```python
from build123d import *

# Parameters (mm, degrees)
SKETCH1_W           = 31.75
SKETCH1_H           = 31.75
BOSS_EXTRUDE1_DEPTH = 114.3
SKETCH3_W           = 24.13
SKETCH3_H           = 24.13
CUT_EXTRUDE1_DEPTH  = 114.3
SKETCH4_W           = 19.05
SKETCH4_H           = 25.4
CUT_EXTRUDE4_DEPTH  = 6.35
SKETCH10_W          = 25.4
SKETCH10_H          = 19.05
CUT_EXTRUDE5_DEPTH  = 6.35
SKETCH13_W          = 19.05
SKETCH13_H          = 25.4
CUT_EXTRUDE6_DEPTH  = 6.35
SKETCH14_W          = 25.4
SKETCH14_H          = 19.05
CUT_EXTRUDE7_DEPTH  = 6.35
FILLET1_64_R        = 0.396875


with BuildPart() as part:
    # Sketch1 → Boss-Extrude1 (new body)
    with BuildSketch(Plane.XY):
        with Locations((-6.389302447, 3.219010904)):
            Rectangle(SKETCH1_W, SKETCH1_H)
    extrude(amount=BOSS_EXTRUDE1_DEPTH)

    # Sketch3 → Cut-Extrude1 (cut)
    with BuildSketch(Plane.XY.offset(114.3)):
        with Locations((-6.389302447, 3.219010904)):
            Rectangle(SKETCH3_W, SKETCH3_H)
    extrude(amount=-CUT_EXTRUDE1_DEPTH, mode=Mode.SUBTRACT)

    # Sketch4 → Cut-Extrude4 (cut)
    with BuildSketch(Plane(origin=(0, 19.094010904, 0), x_dir=(1, 0, 0), z_dir=(0, 1, 0))):
        with Locations((-6.389302447, -76.2)):
            Rectangle(SKETCH4_W, SKETCH4_H)
        with Locations((-6.389302447, -38.1)):
            Rectangle(SKETCH4_W, SKETCH4_H)
    extrude(amount=-CUT_EXTRUDE4_DEPTH, mode=Mode.SUBTRACT)

    # Sketch10 → Cut-Extrude5 (cut)
    with BuildSketch(Plane(origin=(9.485697553, 0, 0), x_dir=(0, 0, -1), z_dir=(1, 0, 0))):
        with Locations((-76.2, 3.219010904)):
            Rectangle(SKETCH10_W, SKETCH10_H)
        with Locations((-38.1, 3.219010904)):
            Rectangle(SKETCH10_W, SKETCH10_H)
    extrude(amount=-CUT_EXTRUDE5_DEPTH, mode=Mode.SUBTRACT)

    # Sketch13 → Cut-Extrude6 (cut)
    with BuildSketch(Plane.XZ.offset(12.655989096)):
        with Locations((-6.389302447, 76.2)):
            Rectangle(SKETCH13_W, SKETCH13_H)
        with Locations((-6.389302447, 38.1)):
            Rectangle(SKETCH13_W, SKETCH13_H)
    extrude(amount=-CUT_EXTRUDE6_DEPTH, mode=Mode.SUBTRACT)

    # Sketch14 → Cut-Extrude7 (cut)
    with BuildSketch(Plane.ZY.offset(22.264302447)):
        with Locations((76.2, 3.219010904)):
            Rectangle(SKETCH14_W, SKETCH14_H)
        with Locations((38.1, 3.219010904)):
            Rectangle(SKETCH14_W, SKETCH14_H)
    extrude(amount=-CUT_EXTRUDE7_DEPTH, mode=Mode.SUBTRACT)

    # Fillet1/64
    fillet1_64_edges = [part.edges().sort_by_distance(p)[0] for p in [
        (-15.914302447, -8.845989096, 38.1),
        (-6.389302447, -8.845989096, 25.4),
        (3.135697553, -8.845989096, 38.1),
        (-6.389302447, -8.845989096, 50.8),
        (-6.389302447, -8.845989096, 63.5),
        (3.135697553, -8.845989096, 76.2),
        (-6.389302447, -8.845989096, 88.9),
        (-15.914302447, -8.845989096, 76.2),
        (-15.914302447, -12.655989096, 76.2),
        (-6.389302447, -12.655989096, 63.5),
        (3.135697553, -12.655989096, 76.2),
        (-6.389302447, -12.655989096, 88.9),
        (9.485697553, 3.219010904, 114.3),
        (-6.389302447, -12.655989096, 50.8),
        (-15.914302447, -12.655989096, 38.1),
        (-6.389302447, -12.655989096, 25.4),
        (3.135697553, -12.655989096, 38.1),
        (-18.454302447, 12.744010904, 38.1),
        (-18.454302447, 3.219010904, 25.4),
        (-18.454302447, -6.305989096, 38.1),
        (-18.454302447, 3.219010904, 50.8),
        (-18.454302447, 3.219010904, 63.5),
        (-18.454302447, -6.305989096, 76.2),
        (-18.454302447, 3.219010904, 88.9),
        (-18.454302447, 12.744010904, 76.2),
        (-22.264302447, 12.744010904, 76.2),
        (-22.264302447, 3.219010904, 63.5),
        (-22.264302447, -6.305989096, 76.2),
        (-22.264302447, 3.219010904, 88.9),
        (-6.389302447, 19.094010904, 114.3),
        (-22.264302447, 3.219010904, 50.8),
        (-22.264302447, 12.744010904, 38.1),
        (-22.264302447, 3.219010904, 25.4),
        (-22.264302447, -6.305989096, 38.1),
        (-6.389302447, -8.845989096, 0),
        (5.675697553, -8.845989096, 57.15),
        (-18.454302447, 3.219010904, 0),
        (-18.454302447, -8.845989096, 57.15),
        (-6.389302447, 15.284010904, 114.3),
        (-18.454302447, 15.284010904, 57.15),
        (5.675697553, 3.219010904, 114.3),
        (5.675697553, 15.284010904, 57.15),
        (-6.389302447, 15.284010904, 0),
        (5.675697553, 3.219010904, 0),
        (-6.389302447, -8.845989096, 114.3),
        (-18.454302447, 3.219010904, 114.3),
        (-6.389302447, 15.284010904, 50.8),
        (3.135697553, 15.284010904, 38.1),
        (-6.389302447, 15.284010904, 25.4),
        (-15.914302447, 15.284010904, 38.1),
        (3.135697553, 15.284010904, 76.2),
        (-6.389302447, 15.284010904, 63.5),
        (-15.914302447, 15.284010904, 76.2),
        (-6.389302447, 15.284010904, 88.9),
        (-15.914302447, 19.094010904, 76.2),
        (-6.389302447, 19.094010904, 63.5),
        (-6.389302447, 19.094010904, 88.9),
        (3.135697553, 19.094010904, 76.2),
        (-6.389302447, 19.094010904, 25.4),
        (3.135697553, 19.094010904, 38.1),
        (-15.914302447, 19.094010904, 38.1),
        (-6.389302447, 19.094010904, 50.8),
        (-22.264302447, 3.219010904, 114.3),
        (-6.389302447, 19.094010904, 0),
        (9.485697553, 3.219010904, 0),
        (-6.389302447, -12.655989096, 0),
        (-22.264302447, 3.219010904, 0),
        (5.675697553, 12.744010904, 38.1),
        (5.675697553, 3.219010904, 50.8),
        (5.675697553, -6.305989096, 38.1),
        (5.675697553, 3.219010904, 25.4),
        (5.675697553, -6.305989096, 76.2),
        (5.675697553, 3.219010904, 63.5),
        (5.675697553, 12.744010904, 76.2),
        (5.675697553, 3.219010904, 88.9),
        (-22.264302447, 19.094010904, 57.15),
        (9.485697553, 12.744010904, 76.2),
        (9.485697553, 19.094010904, 57.15),
        (9.485697553, 3.219010904, 63.5),
        (9.485697553, -12.655989096, 57.15),
        (9.485697553, 3.219010904, 88.9),
        (9.485697553, -6.305989096, 76.2),
        (-22.264302447, -12.655989096, 57.15),
        (9.485697553, 3.219010904, 25.4),
        (9.485697553, -6.305989096, 38.1),
        (-6.389302447, -12.655989096, 114.3),
        (9.485697553, 12.744010904, 38.1),
        (9.485697553, 3.219010904, 50.8),
    ]]
    fillet(fillet1_64_edges, radius=FILLET1_64_R)


solid = part.part
```
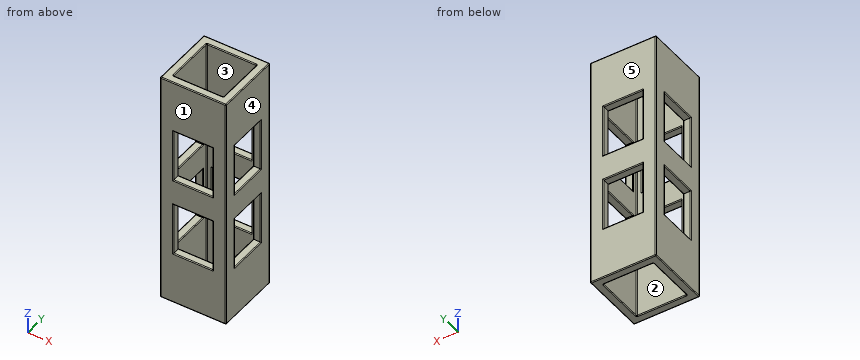
Read the model definition and answer for the solid it produces. Units are mm, in the model's axes. Face numbers are marked on the shaded views. A direction names the side the tool comes from. Round coordinates to 2 decimals unless told otherwise and drop trailing zeros. Write each loop counter-clockwise with the first axis right and the second up, starting at its lowest first coordinate (ties: lowest second). Pieces come first, ordered by that corner, then holes. Notation, with made-up numbers: M -9,-7 L 42,-7 A16 ccw 42,3 Z; hole C 36.25,27.25 d10. An arc over 180 degrees is marked long. One line per item, written item: value.
Q1. Straight lines are drawn through the part: line 1 (Z direction, x = -10, y = -10.5); line 2 (Y direction, x = -18, z = 21); line 3 (X direction, y = 17, z = 75). For each, find the intervals that lie inside material, in ascending order. Write a range as [from, to].
Data:
line 1: [0, 25.4], [50.8, 63.5], [88.9, 114.3]
line 2: [-12.66, -8.85], [15.28, 19.09]
line 3: [-22.26, -15.91], [3.14, 9.49]
Q2. Find section C-C on z = 99. Write down the section's boundary in (x, y).
Data:
outline: M -22.26,-12.26 A0.4 ccw -21.87,-12.66 L 9.09,-12.66 A0.4 ccw 9.49,-12.26 L 9.49,18.7 A0.4 ccw 9.09,19.09 L -21.87,19.09 A0.4 ccw -22.26,18.7 Z; hole M -18.45,-8.45 A0.4 ccw -18.06,-8.85 L 5.28,-8.85 A0.4 ccw 5.68,-8.45 L 5.68,14.89 A0.4 ccw 5.28,15.28 L -18.06,15.28 A0.4 ccw -18.45,14.89 Z
Q3. For a pull along Y with two mould halves and no side action, classify the marked faces 3, 4 and 5 as +Y half, -Y half, draft (parallel to the pull), parting line (faces both ways), or undercut.
Data:
face 3: undercut
face 4: draft
face 5: +Y half
Q4. Which of the six approach directions +Z, -Z, +X, -X, +Y, -Y give full straight-line access (tool end or side, diameter ignored) to the marked faces 1 and 2?
Data:
face 1: +Z, -Z, +X, -X, -Y
face 2: +Z, -Z
Q5. Find section D-D on y = -4.5. Count the separate pieces of the cut face and the enclosed holes in it, plus the area to 3 significant figures.
Data:
separate pieces: 6
enclosed holes: 0
area: 483 mm2
Q6. Find section B-B on y = 17. Write down the section's boundary in (x, z), plus the area to 3 significant figures.
Data:
outline: M -22.26,0.4 A0.4 ccw -21.87,0 L 9.09,0 A0.4 ccw 9.49,0.4 L 9.49,113.9 A0.4 ccw 9.09,114.3 L -21.87,114.3 A0.4 ccw -22.26,113.9 Z; hole M -15.91,25.4 L 3.14,25.4 L 3.14,50.8 L -15.91,50.8 Z; hole M -15.91,63.5 L 3.14,63.5 L 3.14,88.9 L -15.91,88.9 Z
area: 2,660 mm2
Q7. Find section A-A on x = 7.5. Write down the section's boundary in (y, z).
Data:
outline: M -12.66,0.4 A0.4 ccw -12.26,0 L 18.7,0 A0.4 ccw 19.09,0.4 L 19.09,113.9 A0.4 ccw 18.7,114.3 L -12.26,114.3 A0.4 ccw -12.66,113.9 Z; hole M -6.31,25.4 L 12.74,25.4 L 12.74,50.8 L -6.31,50.8 Z; hole M -6.31,63.5 L 12.74,63.5 L 12.74,88.9 L -6.31,88.9 Z
